Autodesk Inventor part; units mm, degrees
ref_plane "YZ Plane" through (0, 0, 0) normal (1, 0, 0) x (0, 1, 0)
ref_plane "XZ Plane" through (0, 0, 0) normal (0, 1, 0) x (-1, 0, 0)
ref_plane "XY Plane" through (0, 0, 0) normal (0, 0, 1) x (1, 0, 0)
sketch "Sketch1" plane through (0, 0, 0) normal (0, 0, 1) x (1, 0, 0)
  line L0 (-52.3875, 0) -> (52.3875, 0) construction
  line L1 (-52.3875, -20.6502) -> (52.3875, -20.6502)
  line L2 (52.3875, 20.6502) -> (-52.3875, 20.6502)
  arc A0 (-52.3875, 20.6502) -> (-52.3875, -20.6502) centre (-52.3875, 0) ccw
  arc A1 (52.3875, -20.6502) -> (52.3875, 20.6502) centre (52.3875, 0) ccw
  point P0 (0, 0)
  dimension "d0" = 104.775
  dimension "d1" = 20.6502
extrude "Extrusion1" add sketch "Sketch1" along normal blind 15.24
sketch "Sketch2" plane through (0, 0, 15.24) normal (0, 0, 1) x (1, 0, 0)
  arc A0 (-52.3875, 20.6502) -> (-52.3875, -20.6502) centre (-52.3875, 0) ccw
  circle A1 centre (-52.3875, 0) radius 14.3002
  arc A2 (52.3875, -20.6502) -> (52.3875, 20.6502) centre (52.3875, 0) ccw
  circle A3 centre (52.3875, 0) radius 14.3002
  point P0 (0, 0)
  dimension "d4" = 28.6004
extrude "Extrusion2" cut sketch "Sketch2" against normal through all
properties part number "IntakeChainLink"
Check sheet for the modelled part. Datum: model origin and axes. Units: mm. Give positions to 0.01 mm unless a question says otherwise; leave off trailing zeros. Order: outer loops, then holes, each group sorted by start corner. A loop starts at its lowest first (then second) coordinate and runs counter-clockwise, first axis right, second up. Notation, with made-up numbers: M 86,45 L 137,45 A15 ccw 137,49 Z; hole C 69,-27 d4. An arc over 180 degrees is marked long. Answer in a Markdown table with one row per item.
1) Cross-section at A-A, the plane y = 0. Enter the section's corners in (x, z), plus the area to 3 significant figures.
Filled sheet:
| item | result |
|---|---|
| outline | M -73.04,0 L -66.69,0 L -66.69,15.24 L -73.04,15.24 Z; M -38.09,0 L 38.09,0 L 38.09,15.24 L -38.09,15.24 Z; M 66.69,0 L 73.04,0 L 73.04,15.24 L 66.69,15.24 Z |
| area | 1,350 mm2 |
2) Release check for a two-part mould opening along X. For faces 1 (the cylindrical face through (-73.033, -0.454, 7.513)), 2 (the cylindrical face through (-63.736, -8.701, 7.727)), 3 (the flat face through (-1, 0, 0)) record: +X half, -X half, draft (parallel to the pull), parting line (faces both ways), or undercut.
Filled sheet:
| item | result |
|---|---|
| face 1 | -X half |
| face 2 | undercut |
| face 3 | draft |
3) Cross-section at B-B, the plane z = 4.5. Enter the section's corners in (x, y).
Filled sheet:
| item | result |
|---|---|
| outline | M -52.39,-20.65 L 52.39,-20.65 A20.65 ccw 52.39,20.65 L -52.39,20.65 A20.65 ccw Z; hole C -52.39,0 d28.6; hole C 52.39,0 d28.6 |
4) Gauge pin test, flat ends, axial feed: P1, Ø4, axis at y = -13.5, z = 9, coming from the +X side; P2, Ø1.5, axis at y = -13, z = 3.5, coming from the +X side. Record the tip position at first contact, or that the pin passes through.
Filled sheet:
| item | result |
|---|---|
| P1 | stops at x = 69.54 |
| P2 | stops at x = 69.01 |
5) Cross-section at D-D, the plane y = 6. Enter the section's corners in (x, z).
Filled sheet:
| item | result |
|---|---|
| outline | M -72.15,0 L -65.37,0 L -65.37,15.24 L -72.15,15.24 Z; M -39.41,0 L 39.41,0 L 39.41,15.24 L -39.41,15.24 Z; M 65.37,0 L 72.15,0 L 72.15,15.24 L 65.37,15.24 Z |
6) Thickness scan on L1, parallel to X at y = 10.5, z = 7.5; L2, parallel to X at y = 12, z = 10.75; L3, parallel to Y at x = 52, z = 14.25. Record the ranges inside material, lowest first. Write a range as [from, to].
Filled sheet:
| item | result |
|---|---|
| L1 | x = [-70.17, -62.1], [-42.68, 42.68], [62.1, 70.17] |
| L2 | x = [-69.19, -60.17], [-44.61, 44.61], [60.17, 69.19] |
| L3 | y = [-20.65, -14.29], [14.29, 20.65] |
7) Cross-section at C-C, the plane x = -42. Enter the section's corners in (y, z), plus the area to 3 significant figures.
Filled sheet:
| item | result |
|---|---|
| outline | M -20.65,0 L -9.83,0 L -9.83,15.24 L -20.65,15.24 Z; M 9.83,0 L 20.65,0 L 20.65,15.24 L 9.83,15.24 Z |
| area | 330 mm2 |
